Autodesk Inventor part; units mm, degrees
ref_plane "WF1_XY" through (0, 7.905, 5.588) normal (1, 0, 0) x (0, 0, -1)
ref_plane "WF1_YZ" through (0, 7.905, 5.588) normal (0, 0, -1) x (0, 1, 0)
ref_plane "WF1_ZX" through (0, 7.905, 5.588) normal (0, 1, 0) x (1, 0, 0)
sketch "Skizze_1" plane through (0, 0, 0) normal (0, 0, 1) x (1, 0, 0)
  arc A0 (1.55, 2.1) -> (3.65, 0) centre (3.65, 2.1) ccw
  line L0 (3.65, 0) -> (12.05, 0)
  line L1 (12.05, 0) -> (12.05, 1.5)
  line L2 (12.05, 1.5) -> (3.65, 1.5)
  arc A1 (3.05, 2.1) -> (3.65, 1.5) centre (3.65, 2.1) ccw
  line L3 (3.05, 2.1) -> (3.05, 10.674)
  line L4 (3.05, 10.674) -> (1.55, 10.674)
  line L5 (1.55, 10.674) -> (1.55, 2.1)
extrude "Extrusion1" add sketch "Skizze_1" along normal blind 23.876
sketch "Skizze_2" plane through (0, 7.905, 0) normal (0, 1, 0) x (1, 0, 0)
  line L0 (-3.8374, -5.588) -> (3.8374, -5.588)
  line L1 (3.8374, -5.588) -> (3.8374, -6.993)
  arc A0 (3.3374, -7.493) -> (3.8374, -6.993) centre (3.3374, -6.993) ccw
  line L2 (3.3374, -7.493) -> (3.05, -7.493)
  line L3 (3.05, -7.493) -> (3.05, -7.1945)
  arc A1 (3.05, -7.1945) -> (2.65, -6.7945) centre (2.65, -7.1945) ccw
  line L4 (2.65, -6.7945) -> (-2.65, -6.7945)
  arc A2 (-2.65, -6.7945) -> (-3.05, -7.1945) centre (-2.65, -7.1945) ccw
  line L5 (-3.05, -7.1945) -> (-3.05, -7.493)
  line L6 (-3.05, -7.493) -> (-3.3374, -7.493)
  arc A3 (-3.8374, -6.993) -> (-3.3374, -7.493) centre (-3.3374, -6.993) ccw
  line L7 (-3.8374, -6.993) -> (-3.8374, -5.588)
  line L8 (-3.8374, -5.588) -> (3.8374, -5.588)
revolve "Revolution1" add sketch "Skizze_2" angle 360 about axis through (-3.8374, 7.905, 5.588) along (-1, 0, 0)
sketch "Skizze_3" plane through (0, 7.905, 0) normal (0, 1, 0) x (1, 0, 0)
  line L0 (-3.8374, -18.288) -> (3.8374, -18.288)
  line L1 (3.8374, -18.288) -> (3.8374, -19.693)
  arc A0 (3.3374, -20.193) -> (3.8374, -19.693) centre (3.3374, -19.693) ccw
  line L2 (3.3374, -20.193) -> (3.05, -20.193)
  line L3 (3.05, -20.193) -> (3.05, -19.8945)
  arc A1 (3.05, -19.8945) -> (2.65, -19.4945) centre (2.65, -19.8945) ccw
  line L4 (2.65, -19.4945) -> (-2.65, -19.4945)
  arc A2 (-2.65, -19.4945) -> (-3.05, -19.8945) centre (-2.65, -19.8945) ccw
  line L5 (-3.05, -19.8945) -> (-3.05, -20.193)
  line L6 (-3.05, -20.193) -> (-3.3374, -20.193)
  arc A3 (-3.8374, -19.693) -> (-3.3374, -20.193) centre (-3.3374, -19.693) ccw
  line L7 (-3.8374, -19.693) -> (-3.8374, -18.288)
  line L8 (-3.8374, -18.288) -> (3.8374, -18.288)
revolve "Revolution2" add sketch "Skizze_3" angle 360 about axis through (-3.8374, 7.905, 18.288) along (-1, 0, 0)
sketch "Skizze_4" plane through (0, 0, 0) normal (0, 0, 1) x (1, 0, 0)
  line L0 (-12.05, 1.5) -> (-12.05, 0)
  line L1 (-12.05, 0) -> (-3.65, 0)
  arc A0 (-3.65, 0) -> (-1.55, 2.1) centre (-3.65, 2.1) ccw
  line L2 (-1.55, 2.1) -> (-1.55, 10.674)
  line L3 (-1.55, 10.674) -> (-3.05, 10.674)
  line L4 (-3.05, 10.674) -> (-3.05, 2.1)
  arc A1 (-3.65, 1.5) -> (-3.05, 2.1) centre (-3.65, 2.1) ccw
  line L5 (-3.65, 1.5) -> (-12.05, 1.5)
extrude "Extrusion2" add sketch "Skizze_4" along normal blind 23.876
sketch "Skizze_5" plane through (0, 0, 0) normal (1, 0, 0) x (0, 1, 0)
  line L0 (-7, 30) -> (-7, -7)
  line L1 (-7, -7) -> (15, -7)
  line L2 (15, -7) -> (15, 30)
  line L3 (15, 30) -> (-7, 30)
  line L4 (1.5, 23.876) -> (0, 23.876)
  line L5 (0, 23.876) -> (0, 0)
  line L6 (0, 0) -> (1.5, 0)
  line L7 (1.5, 0) -> (9.029, 3.0378)
  arc A0 (9.029, 3.0378) -> (8, 8.338) centre (8, 5.588) ccw
  arc A1 (4.4, 11.938) -> (8, 8.338) centre (8, 11.938) ccw
  arc A2 (8, 15.538) -> (4.4, 11.938) centre (8, 11.938) ccw
  arc A3 (8, 15.538) -> (9.029, 20.8382) centre (8, 18.288) ccw
  line L8 (9.029, 20.8382) -> (1.5, 23.876)
extrude "Extrusion3" cut sketch "Skizze_5" along normal mid plane 50
sketch "Skizze_6" plane through (0, 0, 0) normal (0, 1, 0) x (-1, 0, 0)
  line L0 (31, 46) -> (-49, 46)
  line L1 (-49, 46) -> (-49, -17)
  line L2 (-49, -17) -> (31, -17)
  line L3 (31, -17) -> (31, 46)
  arc A0 (12.05, 20.876) -> (9.05, 23.876) centre (9.05, 20.876) ccw
  line L4 (9.05, 23.876) -> (-9.05, 23.876)
  arc A1 (-9.05, 23.876) -> (-12.05, 20.876) centre (-9.05, 20.876) ccw
  line L5 (-12.05, 20.876) -> (-12.05, 3)
  arc A2 (-12.05, 3) -> (-9.05, 0) centre (-9.05, 3) ccw
  line L6 (-9.05, 0) -> (9.05, 0)
  arc A3 (9.05, 0) -> (12.05, 3) centre (9.05, 3) ccw
  line L7 (12.05, 3) -> (12.05, 20.876)
extrude "Extrusion4" cut sketch "Skizze_6" along normal blind 5
sketch "Skizze_7" plane through (0, 0, 0) normal (0, 1, 0) x (-1, 0, 0)
  arc A0 (-5.827, 6.337) -> (-10.1958, 6.337) centre (-8.0114, 6.337) ccw
  line L0 (-10.1958, 6.337) -> (-10.1958, 3.937)
  arc A1 (-10.1958, 3.937) -> (-5.827, 3.937) centre (-8.0114, 3.937) ccw
  line L1 (-5.827, 3.937) -> (-5.827, 6.337)
extrude "Extrusion5" cut sketch "Skizze_7" along normal blind 1.5
sketch "Skizze_8" plane through (0, 0, 0) normal (0, 1, 0) x (-1, 0, 0)
  line L0 (-5.827, 17.539) -> (-5.827, 19.939)
  arc A0 (-5.827, 19.939) -> (-10.1958, 19.939) centre (-8.0114, 19.939) ccw
  line L1 (-10.1958, 19.939) -> (-10.1958, 17.539)
  arc A1 (-10.1958, 17.539) -> (-5.827, 17.539) centre (-8.0114, 17.539) ccw
extrude "Extrusion6" cut sketch "Skizze_8" along normal blind 5
sketch "Skizze_10" plane through (0, 0, 0) normal (0, 1, 0) x (-1, 0, 0)
  arc A0 (10.1958, 6.337) -> (5.827, 6.337) centre (8.0114, 6.337) ccw
  line L0 (5.827, 6.337) -> (5.827, 3.937)
  arc A1 (5.827, 3.937) -> (10.1958, 3.937) centre (8.0114, 3.937) ccw
  line L1 (10.1958, 3.937) -> (10.1958, 6.337)
extrude "Extrusion7" cut sketch "Skizze_10" along normal blind 5
sketch "Skizze_11" plane through (0, 0, 0) normal (0, 1, 0) x (-1, 0, 0)
  line L0 (10.1958, 17.539) -> (10.1958, 19.939)
  arc A0 (10.1958, 19.939) -> (5.827, 19.939) centre (8.0114, 19.939) ccw
  line L1 (5.827, 19.939) -> (5.827, 17.539)
  arc A1 (5.827, 17.539) -> (10.1958, 17.539) centre (8.0114, 17.539) ccw
extrude "Extrusion8" cut sketch "Skizze_11" along normal blind 3
ref_plane "WF1_XY" through (0, 7.905, 5.588) normal (1, 0, 0) x (0, 0, -1)
ref_plane "WF1_YZ" through (0, 7.905, 5.588) normal (0, 0, -1) x (0, 1, 0)
ref_plane "WF1_ZX" through (0, 7.905, 5.588) normal (0, 1, 0) x (1, 0, 0)
ref_plane "WF2_XY" through (0, 7.905, 18.288) normal (1, 0, 0) x (0, 0, -1)
ref_plane "WF2_YZ" through (0, 7.905, 18.288) normal (0, 0, -1) x (0, 1, 0)
ref_plane "WF2_ZX" through (0, 7.905, 18.288) normal (0, 1, 0) x (1, 0, 0)
properties part number "205-S-WF"
Can you work these out from the model? Positions are in its coordinate system, mm. A direction names the side the tool comes from. Give positions to 0.01 mm unless a question says otherwise; leave off trailing zeros. Order: outer loops, then holes, each group sorted by start corner. A loop starts at its lowest first (then second) coordinate and runs counter-clockwise, first axis right, second up. Notation, with made-up numbers: M 4,76.25 L 26,76.25 A11 cw 26,88.25 Z; hole C -2.75,81 d10. An arc over 180 degrees is marked long. One line per item, written item: value.
Item 1: If we section it at B-B on y = 2.5: Write out the boundary of the cut face in (x, z).
Verdict:
outline: M -3.05,0.4 L -1.55,0.4 L -1.55,23.47 L -3.05,23.47 Z; M 1.55,0.4 L 3.05,0.4 L 3.05,23.47 L 1.55,23.47 Z
Item 2: Please list where these lines run through material, in increasing order: line 1 (X direction, y = 5.25, z = 21.75); line 2 (X direction, y = 0.5, z = 16.75); line 3 (Y direction, x = 5, z = 3.75).
Verdict:
line 1: -3.05 to -1.55, 1.55 to 3.05
line 2: -12.05 to -10.05, -5.97 to -2.29, 2.29 to 5.97, 10.05 to 12.05
line 3: 0 to 1.5
Item 3: If we section it at A-A on z = 9.5: Write out the boundary of the cut face in (x, y), and give its area (3 significant figures).
Verdict:
outline: M -12.05,0 L -3.65,0 A2.1 ccw -1.55,2.1 L -1.55,5.35 L -3.05,5.35 L -3.05,2.1 A0.6 cw -3.65,1.5 L -12.05,1.5 Z; M 1.55,2.1 A2.1 ccw 3.65,0 L 12.05,0 L 12.05,1.5 L 3.65,1.5 A0.6 cw 3.05,2.1 L 3.05,5.35 L 1.55,5.35 Z
area: 41.3 mm2
Item 4: For faces 1 (the face through (-11.19, 0.74, 0.9)), 2 (the face through (10.196, 1, 5)), 3 (the face through (-0.022, 7.958, 17.083)), which set-ups out of +Z, -Z, +X, -X, +Y, -Y let a thin tool reach every point of the face, with its end or its side?
Verdict:
face 1: -Z, -X, +Y, -Y
face 2: +Y, -Y
face 3: none
Item 5: If we section it at D-D on x = -1: Write out the boundary of the cut face in (y, z) (1 decimal).
Verdict:
outline: C 7.9,5.6 d2.4; C 7.9,18.3 d2.4
Item 6: If we section it at C-C on x = 9.75: Write out the boundary of the cut face in (y, z).
Verdict:
outline: M 0,0.08 L 1.5,0.08 L 1.5,2.61 L 0,2.61 Z; M 0,7.66 L 1.5,7.66 L 1.5,16.22 L 0,16.22 Z; M 0,21.26 L 1.5,21.26 L 1.5,23.79 L 0,23.79 Z
Item 7: For pin 1 (0.8 mm diameter, centred on y = 7.5, z = 18, fed in from +X); pin 2 (6 mm diameter, centred on x = -9.5, y = 8.5, fed in from +Z); pin 3 (2 mm diameter, centred on y = 8, z = 18.5, fed in from -X); pin 4 (2.5 mm diameter, centred on x = 6.5, z = 8, fed in from +Y), each with a flat end and sliding along its axis, tell me the tip position at first contact or that it passes through.
Verdict:
pin 1: x = 3.84
pin 2: through
pin 3: x = -3.84
pin 4: y = 1.5
